Answer from the drawing. Dimensions are ordinates in mm from the lowest x, y and z of the part. Round coordinates to 2 decimals unless told otherwise and drop trailing zeros. Order: outer loops, then holes, each group sorted by start corner. A loop starts at its lowest first (then second) coordinate and runs counter-clockwise, first axis right, second up. Notation, with made-up numbers: M 28.25,53.25 L 80.25,53.25 A35 ccw 80.25,87.25 Z; hole C -11.5,79.5 d6. An arc over 180 degrees is marked long. Write item = value, one per line. Start each with the question number.
(1) Straight lines are drawn through the part: probe 1 along X at (y, z) = (1.75, 55) (1 decimal); probe 2 along X at (y, z) = (2.2, 45); probe 3 along Z at (x, y) = (10, 2.25). For each, find the intervals that lie inside material, in ascending order. Write a range as from..to.
(2) A cutting plane is placed at A-A, the plane z = 32.5. Determine the outline of the cut face in (x, y) (1 decimal).
(3) A cutting plane is placed at B-B, the plane y = 1.45. Determine the outline of the cut face in (x, z) (1 decimal).
(4) This flat-tipped pin is pushed along its axis until it touches: pin 1 (0.5 mm diameter, centred on x = 8, y = 1.5, fed in from +Z). Where does it stop, or does it pass through?
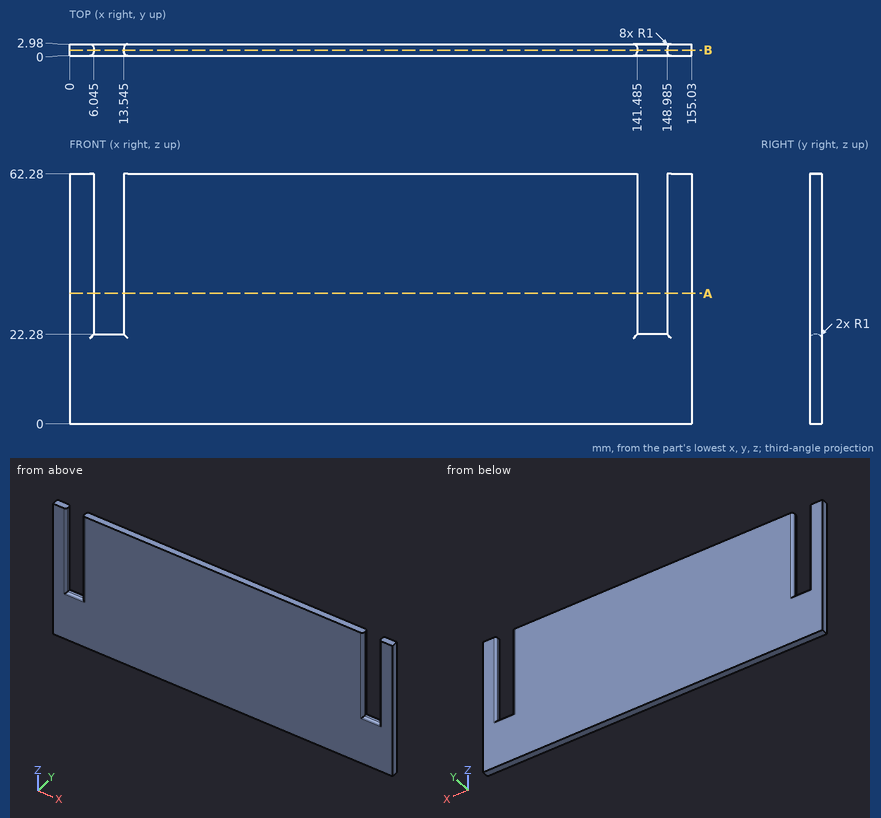
Reported:
q1.probe_1 = 0..6, 13.5..141.5, 149..155
q1.probe_2 = 0..6.02, 13.57..141.46, 149.01..155.03
q1.probe_3 = 0..22.24
q2.outline = M 0,0 L 5,0 A1 ccw 6,1 L 6,2 A1 ccw 5,3 L 0,3 Z; M 13.5,1 A1 ccw 14.5,0 L 140.5,0 A1 ccw 141.5,1 L 141.5,2 A1 ccw 140.5,3 L 14.5,3 A1 ccw 13.5,2 Z; M 149,1 A1 ccw 150,0 L 155,0 L 155,3 L 150,3 A1 ccw 149,2 Z
q3.outline = M 0,0 L 155,0 L 155,62.3 L 149,62.3 L 149,22.3 L 141.5,22.3 L 141.5,62.3 L 13.5,62.3 L 13.5,22.3 L 6,22.3 L 6,62.3 L 0,62.3 Z
q4.pin_1 = 22.28
